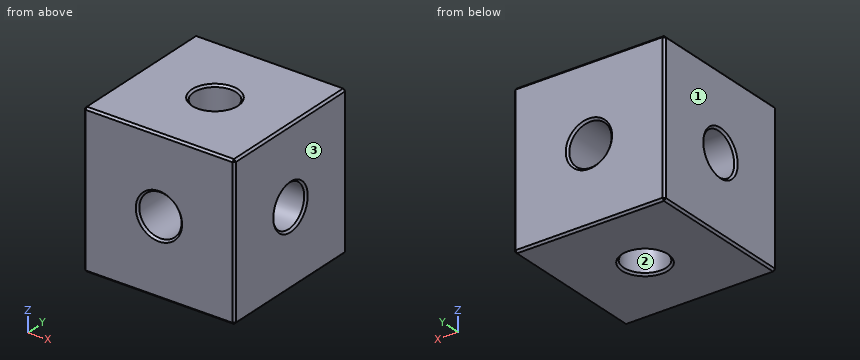
from build123d import *

# Parameters (mm, degrees)
SKETCH_1_W         = 15
SKETCH_1_H         = 15
EXTRUDE_1_DEPTH    = 7.5
HOLE_WIZARD_M5_1_D = 4.2
HOLE_WIZARD_M5_2_D = 4.2
HOLE_WIZARD_M5_3_D = 4.2
CHAMFER_1_SIZE     = 0.2


with BuildPart() as part:
    # 草图1 → 凸台-拉伸1 (new, symmetric)
    with BuildSketch(Plane(origin=(0, 0, 0), x_dir=(1, 0, 0), z_dir=(0, 1, 0))):
        Rectangle(SKETCH_1_W, SKETCH_1_H)
    extrude(amount=EXTRUDE_1_DEPTH, both=True)

    # M5 螺纹孔1 (through all)
    with Locations(Plane.XY.offset(7.5)):
        with Locations((0, 0)):
            Hole(HOLE_WIZARD_M5_1_D / 2)

    # M5 螺纹孔2 (through all)
    with Locations(Plane(origin=(0, 7.5, 0), x_dir=(1, 0, 0), z_dir=(0, 1, 0))):
        with Locations((0, 0)):
            Hole(HOLE_WIZARD_M5_2_D / 2)

    # M5 螺纹孔3 (through all)
    with Locations(Plane(origin=(7.5, 0, 0), x_dir=(0, 0, -1), z_dir=(1, 0, 0))):
        with Locations((0, 0)):
            Hole(HOLE_WIZARD_M5_3_D / 2)

    # 倒角1
    chamfer_1_edges = [part.edges().sort_by_distance(p)[0] for p in [
        (-7.5, 7.5, 0),
        (2.1, 0, 7.5),
        (2.1, 0, -7.5),
        (0, 7.5, 7.5),
        (2.1, -7.5, 0),
        (2.1, 7.5, 0),
        (-7.5, 0, -2.1),
        (7.5, 0, -2.1),
        (7.5, 7.5, 0),
        (0, -7.5, 7.5),
        (-7.5, -7.5, 0),
        (0, -7.5, -7.5),
        (7.5, -7.5, 0),
        (7.5, 0, 7.5),
        (-7.5, 0, 7.5),
        (-7.5, 0, -7.5),
        (7.5, 0, -7.5),
        (0, 7.5, -7.5),
    ]]
    chamfer(chamfer_1_edges, length=CHAMFER_1_SIZE)


solid = part.part
Input: part model. Units: mm. Frame: model coordinates. Face numbers are marked on the shaded views. Coordinates: 2 decimals unless noted, no trailing zeros. Order: outer loops, then holes, each group sorted by start corner. A loop starts at its lowest first (then second) coordinate and runs counter-clockwise, first axis right, second up.
1. Cut plane C-C, the plane x = -2.75. Return loops of the section in (y, z).
Checked values:
outline: (-7.5, -7.3) - (-7.3, -7.5) - (7.3, -7.5) - (7.5, -7.3) - (7.5, 7.3) - (7.3, 7.5) - (-7.3, 7.5) - (-7.5, 7.3) - close; hole circle Ø4.2 at (0, 0)
2. Cut plane A-A, the plane y = 0. Return loops of the section in (x, z).
Checked values:
outline: (-7.5, -7.3) - (-7.3, -7.5) - (-2.3, -7.5) - (-2.1, -7.3) - (-2.1, -2.1) - (-7.3, -2.1) - (-7.5, -2.3) - close; (-7.5, 2.3) - (-7.3, 2.1) - (-2.1, 2.1) - (-2.1, 7.3) - (-2.3, 7.5) - (-7.3, 7.5) - (-7.5, 7.3) - close; (2.1, -7.3) - (2.3, -7.5) - (7.3, -7.5) - (7.5, -7.3) - (7.5, -2.3) - (7.3, -2.1) - (2.1, -2.1) - close; (2.1, 2.1) - (7.3, 2.1) - (7.5, 2.3) - (7.5, 7.3) - (7.3, 7.5) - (2.3, 7.5) - (2.1, 7.3) - close
3. Ray query, line 1 along Y through (x, z) = (0, 3.6). Return the intervals inside material, ascending.
Checked values:
line 1: y = -7.5 to -2.1, 2.1 to 7.5
4. Contact query for a flat-ended pin moving along its axis: P1, Ø4, axis at x = 0, z = 0, coming from the +Y side. Output: stop coordinate, or through.
Checked values:
P1: passes through
5. Draft query along X for the marked faces 1, 2 and 3. Return one class per face: +X half, -X half, draft (parallel to the pull), parting line (faces both ways), or undercut.
Checked values:
face 1: -X half
face 2: undercut
face 3: +X half
